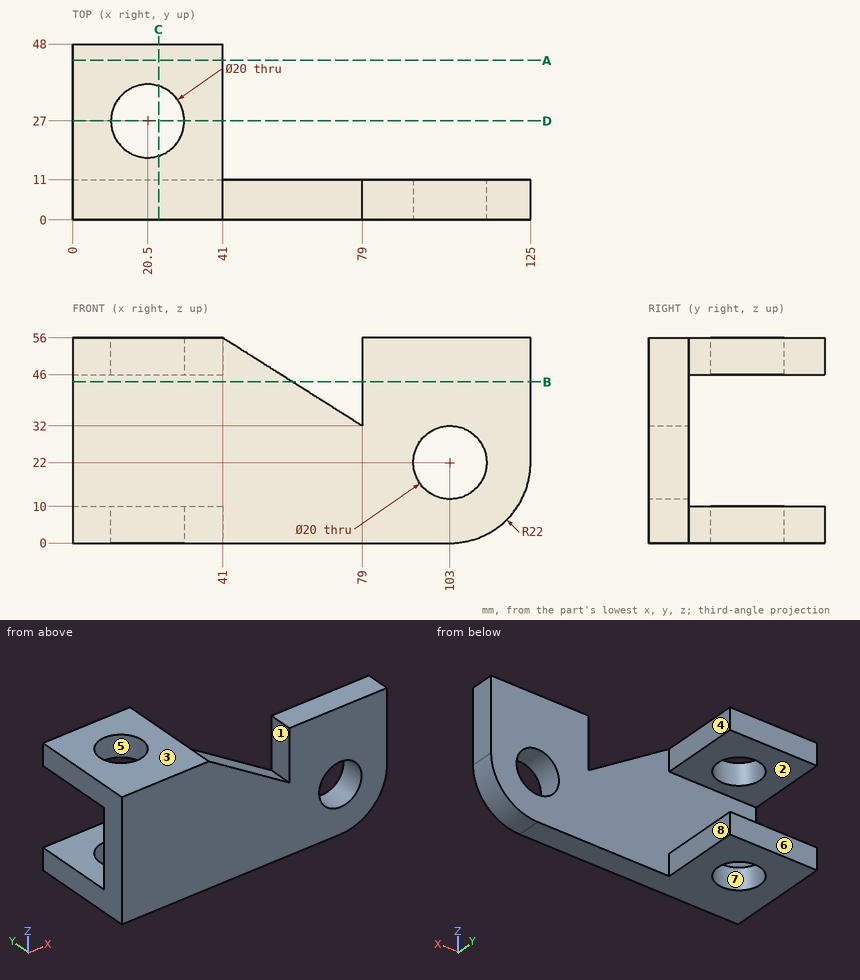
Geometry: see drawing. Coordinates: mm, zero at the bounding-box minimum. A direction names the side the tool comes from. Coordinates: 2 decimals unless noted, no trailing zeros. Loops run counter-clockwise (first coordinate to the right, second up) from the corner with the lowest first, then second, coordinate; pieces in that order, holes last. Notation, with made-up numbers: (-5, 9.25) - (4, 9.25) arc R23 ccw to (4, 48.25) - close; hole circle Ø3 at (-4, 35). An arc over 180 degrees is marked (long way). Answer in a Markdown table with one row per item.
(1) Material intervals for L1, parallel to X at y = 4.25, z = 22; L2, parallel to Z at x = 13.5, y = 19.5; L3, parallel to Z at x = 103, y = 9.25, sorted ascending. Write a range as from..to.
Model answer:
| item | result |
|---|---|
| L1 | x = 0..93, 113..125 |
| L2 | z = 0..10, 46..56 |
| L3 | z = 0..12, 32..56 |
(2) Cut plane C-C on x = 23.5. Output: boundary loops of the cut face in (y, z), plus the area to 3 significant figures.
Model answer:
| item | result |
|---|---|
| outline | (0, 0) - (17.46, 0) - (17.46, 10) - (11, 10) - (11, 46) - (17.46, 46) - (17.46, 56) - (0, 56) - close; (36.54, 0) - (48, 0) - (48, 10) - (36.54, 10) - close; (36.54, 46) - (48, 46) - (48, 56) - (36.54, 56) - close |
| area | 974 mm² |
(3) Cut plane B-B on z = 44. Output: boundary loops of the cut face in (x, y).
Model answer:
| item | result |
|---|---|
| outline | (0, 0) - (60, 0) - (60, 11) - (0, 11) - close; (79, 0) - (125, 0) - (125, 11) - (79, 11) - close |
(4) Pin query (flat end, axial travel): P1, Ø3, axis at y = 26, z = 5.5, coming from the +X side; P2, Ø12, axis at y = 22, z = 28.5, coming from the +X side; P3, Ø3, axis at y = 11, z = 13, coming from the +X side. Return the tip coordinate at first contact, or that it passes through.
Model answer:
| item | result |
|---|---|
| P1 | stops at x = 41 |
| P2 | passes through |
| P3 | stops at x = 123.68 |
(5) Set-up query: the marked faces 1, 2, 3 and 4. Return all of +Z, -Z, +X, -X, +Y, -Y with unobstructed straight access to the full face (end or side cutting, diameter ignored); none if empty.
Model answer:
| item | result |
|---|---|
| face 1 | +Z, +Y, -Y |
| face 2 | +X, -X, +Y |
| face 3 | +Z, +X, -X, +Y, -Y |
| face 4 | +Z, -Z, +X, +Y |
(6) Cut plane D-D on y = 27. Output: boundary loops of the cut face in (x, z).
Model answer:
| item | result |
|---|---|
| outline | (0, 0) - (10.5, 0) - (10.5, 10) - (0, 10) - close; (0, 46) - (10.5, 46) - (10.5, 56) - (0, 56) - close; (30.5, 0) - (41, 0) - (41, 10) - (30.5, 10) - close; (30.5, 46) - (41, 46) - (41, 56) - (30.5, 56) - close |
(7) Cut plane A-A on y = 43.5. Output: boundary loops of the cut face in (x, z), plus the area to 3 significant figures.
Model answer:
| item | result |
|---|---|
| outline | (0, 0) - (41, 0) - (41, 10) - (0, 10) - close; (0, 46) - (41, 46) - (41, 56) - (0, 56) - close |
| area | 820 mm² |
(8) Mould query, pull axis Y, two halves, no side actions, for the marked faces 5, 6, 7 and 8. Classes: pulls with the +Y half, pulls with the -Y half, needs draft (parallel to the pull), parting line crosses it, or undercut.
Model answer:
| item | result |
|---|---|
| face 5 | undercut |
| face 6 | pulls with the +Y half |
| face 7 | undercut |
| face 8 | needs draft |
